```python
from build123d import *

# Parameters (mm, degrees)
SKETCH1_W                        = 25.4
SKETCH1_H                        = 50.8
SKETCH1_W_2                      = 19.05
SKETCH1_H_2                      = 44.45
BOSS_EXTRUDE1_DEPTH              = 152.4
SKETCH2_R                        = 2.4638
CUT_EXTRUDE1_DEPTH               = 163.639355631
F_13_64_0_20313_DIAMETER_HOLE1_D = 5.159502


with BuildPart() as part:
    # Sketch1 → Boss-Extrude1 (new body)
    with BuildSketch(Plane(origin=(0, 0, 0), x_dir=(1, 0, 0), z_dir=(0, 1, 0))):
        with Locations((12.7, 25.4)):
            Rectangle(SKETCH1_W, SKETCH1_H)
        with Locations((12.7, 25.4)):
            Rectangle(SKETCH1_W_2, SKETCH1_H_2, mode=Mode.SUBTRACT)
    extrude(amount=BOSS_EXTRUDE1_DEPTH)

    # Sketch2 → Cut-Extrude1 (cut, through all)
    with BuildSketch(Plane.XY):
        with Locations((12.7, 82.55)):
            Circle(SKETCH2_R)
        with Locations((12.7, 57.15)):
            Circle(SKETCH2_R)
        with Locations((12.7, 19.05)):
            Circle(SKETCH2_R)
    extrude(amount=-CUT_EXTRUDE1_DEPTH, mode=Mode.SUBTRACT)

    # 13/64 (0.20313) Diameter Hole1 (through all)
    with Locations(Plane.ZY):
        with Locations((-34.925, 123.822021436), (-15.875, 123.822021436)):
            Hole(F_13_64_0_20313_DIAMETER_HOLE1_D / 2)


solid = part.part
```
The model under review builds one solid part; all positions refer to its coordinate system, in mm. A direction names the side the tool comes from. Give positions to 0.01 mm unless a question says otherwise; leave off trailing zeros. Write each loop counter-clockwise with the first axis right and the second up, starting at its lowest first coordinate (ties: lowest second). Pieces come first, ordered by that corner, then holes. Notation, with made-up numbers: M -38.5,44.25 L -3.5,44.25 A29 cw -3.5,82.25 Z; hole C 26,-37.75 d6. An arc over 180 degrees is marked long. Answer in a Markdown table with one row per item.
Item 1: Add section B-B on x = 7.75. Give the boundary of the cut face in (y, z) (3 decimals), plus the area to 3 significant figures.
Check sheet entries:
| item | result |
|---|---|
| outline | M 0,-50.8 L 152.4,-50.8 L 152.4,-47.625 L 0,-47.625 Z; M 0,-3.175 L 152.4,-3.175 L 152.4,0 L 0,0 Z |
| area | 968 mm2 |
Item 2: Add section C-C on z = -39. Give the boundary of the cut face in (x, y) (3 decimals), plus the area to 3 significant figures.
Check sheet entries:
| item | result |
|---|---|
| outline | M 0,0 L 3.175,0 L 3.175,152.4 L 0,152.4 Z; M 22.225,0 L 25.4,0 L 25.4,152.4 L 22.225,152.4 Z |
| area | 968 mm2 |
Item 3: Draft analysis for pull direction X (two halves, no side actions). For faces 1 (the face through (0, 75, -25)), 2 (the face through (13, 75, 0)), 3 (the face through (10.745, 17.551, -1.565)), 4 (the face through (13, 75, -47.625)), state which applies: +X half, -X half, draft (parallel to the pull), parting line (faces both ways), or undercut.
Check sheet entries:
| item | result |
|---|---|
| face 1 | -X half |
| face 2 | draft |
| face 3 | undercut |
| face 4 | undercut |
Item 4: Tool access review of faces 5 (the face through (2, 0, -24)), 6 (the face through (3.175, 75, -25)): name each direction out of +Z, -Z, +X, -X, +Y, -Y from which nothing blocks a thin tool from reaching the whole face with its end or side.
Check sheet entries:
| item | result |
|---|---|
| face 5 | +Z, -Z, +X, -X, -Y |
| face 6 | +Y, -Y |
Item 5: For line 1 along Y through (x, z) = (12.7, -1); line 2 along X through (y, z) = (32.5, -9.5) (3 decimals); line 3 along Z through (x, y) = (20.25, 78) (3 decimals), list the stretches that pass through material, from the lowest coordinate up.
Check sheet entries:
| item | result |
|---|---|
| line 1 | 0 to 16.59, 21.51 to 54.69, 59.61 to 80.09, 85.01 to 152.4 |
| line 2 | 0 to 3.175, 22.225 to 25.4 |
| line 3 | -50.8 to -47.625, -3.175 to 0 |
Item 6: Add section A-A on y = 57.15. Give the boundary of the cut face in (x, z) (3 decimals), plus the area to 3 significant figures.
Check sheet entries:
| item | result |
|---|---|
| outline | M 0,-50.8 L 10.236,-50.8 L 10.236,-47.625 L 3.175,-47.625 L 3.175,-3.175 L 10.236,-3.175 L 10.236,0 L 0,0 Z; M 15.164,-50.8 L 25.4,-50.8 L 25.4,0 L 15.164,0 L 15.164,-3.175 L 22.225,-3.175 L 22.225,-47.625 L 15.164,-47.625 Z |
| area | 412 mm2 |
Item 7: Add section D-D on y = 111.5. Give the boundary of the cut face in (x, z) (3 decimals).
Check sheet entries:
| item | result |
|---|---|
| outline | M 0,-50.8 L 25.4,-50.8 L 25.4,0 L 0,0 Z; hole M 3.175,-47.625 L 22.225,-47.625 L 22.225,-3.175 L 3.175,-3.175 Z |
